Could you check a few things on this drawing? It's one solid part, dimensions in mm from its lowest x, y, z. Round coordinates to 2 decimals unless told otherwise and drop trailing zeros. Write each loop counter-clockwise with the first axis right and the second up, starting at its lowest first coordinate (ties: lowest second). Pieces come first, ordered by that corner, then holes. Notation, with made-up numbers: (38.5, 7.5) -> (44.5, 7.5) arc R33 cw to (44.5, 44.5) -> close; hole circle Ø7 at (25, -25). An arc over 180 degrees is marked (long way). Answer in a Markdown table with one row per item.
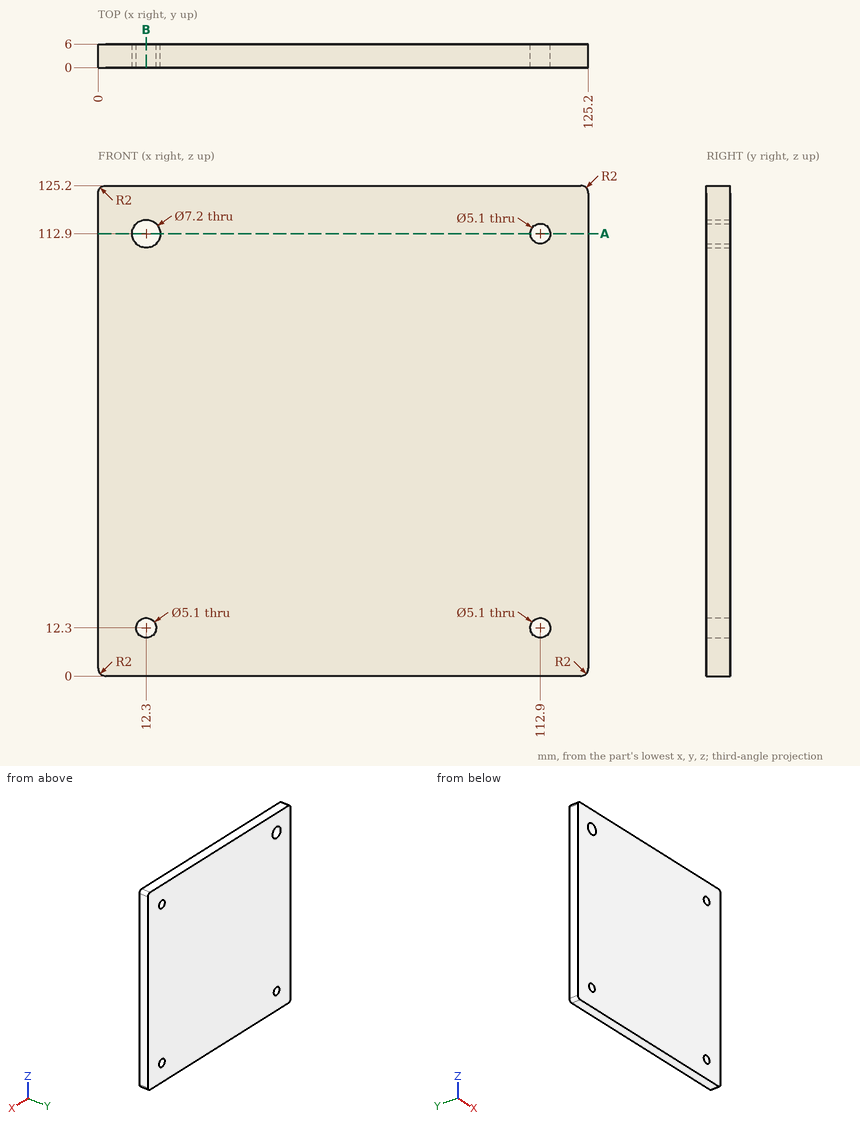
1) I need wall thicknesses on line 1 (X direction, y = 4.2, z = 112.9); line 2 (Z direction, x = 112.9, y = 3.2); line 3 (Z direction, x = 12.3, y = 4.8). Which ranges of each line are inside material? Lowest first, please. Write a range as [from, to].
Response:
| item | result |
|---|---|
| line 1 | x = [0, 8.7], [15.9, 110.35], [115.45, 125.2] |
| line 2 | z = [0, 9.75], [14.85, 110.35], [115.45, 125.2] |
| line 3 | z = [0, 9.75], [14.85, 109.3], [116.5, 125.2] |
2) For pin 1 (3 mm diameter, centred on x = 12.3, z = 12.3, fed in from +Y), with a flat end and sliding along its axis, tell me the tip position at first contact or that it passes through.
Response:
| item | result |
|---|---|
| pin 1 | passes through |
3) I want a section at A-A, the plane z = 112.9. List the corners of the cut face in (x, y) for me, and give its area (3 significant figures).
Response:
| item | result |
|---|---|
| outline | (0, 0) -> (8.7, 0) -> (8.7, 6) -> (0, 6) -> close; (15.9, 0) -> (110.35, 0) -> (110.35, 6) -> (15.9, 6) -> close; (115.45, 0) -> (125.2, 0) -> (125.2, 6) -> (115.45, 6) -> close |
| area | 677 mm^2 |
4) I want a section at B-B, the plane x = 12.3. List the corners of the cut face in (y, z) for me, and give its area (3 significant figures).
Response:
| item | result |
|---|---|
| outline | (0, 0) -> (6, 0) -> (6, 9.75) -> (0, 9.75) -> close; (0, 14.85) -> (6, 14.85) -> (6, 109.3) -> (0, 109.3) -> close; (0, 116.5) -> (6, 116.5) -> (6, 125.2) -> (0, 125.2) -> close |
| area | 677 mm^2 |
